from build123d import *

# Parameters (mm, degrees)
SKETCH004_R       = 5.031
PAD005_DEPTH      = 15
SKETCH007_W       = 23.03
SKETCH007_H       = 7
POCKET_DEPTH      = 9.031
POCKET_DEPTH_BACK = 9.031
SKETCH008_W       = 20
SKETCH008_H       = 23
PAD006_DEPTH      = 2
PAD012_DEPTH      = 4
PAD013_DEPTH      = 19


with BuildPart() as part:
    # Sketch004 → Pad005 (new body)
    with BuildSketch(Plane.XY):
        with BuildLine():
            ThreePointArc((-9.03, 0), (0, -9.03), (9.03, 0))
            Line((9.03, 0), (9.03, 16))
            Line((9.03, 16), (-9.03, 16))
            Line((-9.03, 16), (-9.03, 0))
        make_face()
        Circle(SKETCH004_R, mode=Mode.SUBTRACT)
    extrude(amount=PAD005_DEPTH)

    # Sketch007 → Pocket (cut, two sides)
    with BuildSketch(Plane.YZ) as pocket_sk:
        with Locations((2.485, 7.5)):
            Rectangle(SKETCH007_W, SKETCH007_H)
    extrude(amount=-POCKET_DEPTH, mode=Mode.SUBTRACT)
    extrude(pocket_sk.sketch, amount=POCKET_DEPTH_BACK, mode=Mode.SUBTRACT)

    # Sketch008 → Pad006 (join)
    with BuildSketch(Plane.XZ.offset(-16)):
        with Locations((10, 7.5)):
            Rectangle(SKETCH008_W, SKETCH008_H)
    extrude(amount=PAD006_DEPTH)

    # Sketch018 → Pad012 (join)
    with BuildSketch(Plane.XY):
        Polygon((14, 16.280637), (14, -8), (26, -8), (26, -4.5), (24, -4.5), (24, -6), (16, -6), (16, 14), (54, 14), (54, 12), (56, 12), (56, 14), (56, 16), (14, 16), align=None)
    extrude(amount=-PAD012_DEPTH)

    # Sketch018 → Pad013 (join)
    with BuildSketch(Plane.XY):
        Polygon((14, 16.280637), (14, -8), (26, -8), (26, -4.5), (24, -4.5), (24, -6), (16, -6), (16, 14), (54, 14), (54, 12), (56, 12), (56, 14), (56, 16), (14, 16), align=None)
    extrude(amount=PAD013_DEPTH)


solid = part.part
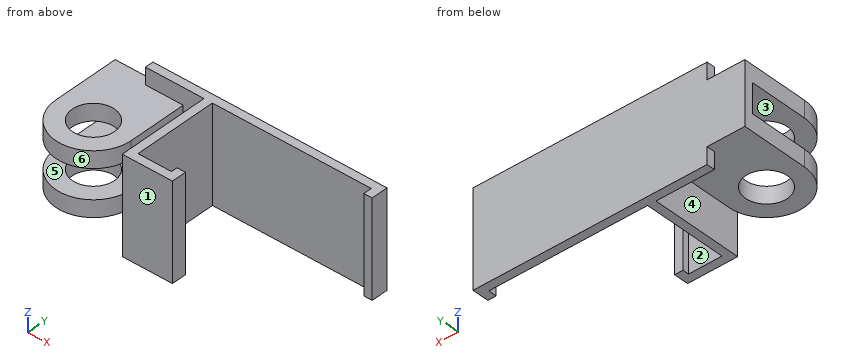
Check sheet for the modelled part. Datum: model origin and axes. Units: mm. Face numbers are marked on the shaded views. A direction names the side the tool comes from. Round coordinates to 2 decimals unless told otherwise and drop trailing zeros. Order: outer loops, then holes, each group sorted by start corner. A loop starts at its lowest first (then second) coordinate and runs counter-clockwise, first axis right, second up. Notation, with made-up numbers: M 63.5,-15.75 L 115.5,-15.75 A16 cw 115.5,-6.75 Z; hole C 6.25,22 d9. An arc over 180 degrees is marked long. One line per item, written item: value. Start each with the question number.
1. Section check D-D on x = 47.5. Enter the section's corners in (y, z), and give its area (3 significant figures).
2. Gauge pin test, flat ends, axial feed: P1, Ø1.6, axis at y = 15, z = -1.5, coming from the -X side; P2, Ø4, axis at y = -6.5, z = 10, coming from the +X side; P3, Ø14.5, axis at x = -3.5, y = 7, coming from the +Z side. Record the tip position at first contact, or that the pin passes through.
3. Scan lines: line 1 along X through (y, z) = (11, 12.5); line 2 along Y through (x, z) = (0, 12.15); line 3 along X through (y, z) = (0.75, 12). Record each from-to range of solid material in increasing order.
4. Access from +Z, -Z, +X, -X, +Y, -Y to the whole of each face (thin tool, end or side, straight path). Record for the marked faces 1, 2 and 3.
5. Section check C-C on y = -1. Enter the section's corners in (x, z).
6. Section check B-B on z = 14. Enter the section's corners in (x, y).
7. Release check for a two-part mould opening along X. For the marked faces 4, 5 and 6 record: released by +X, released by -X, zero draft, split by the parting line, or undercut.
8. Section check A-A on z = 7.5. Enter the section's corners in (x, y).
Results found:
1. outline: M 14,-4 L 16,-4 L 16,19 L 14,19 Z
1. area: 46.0 mm^2
2. P1: x = 0
2. P2: x = 26
2. P3: z = 15
3. line 1: -9.03 to 9.03, 14 to 16
3. line 2: -9.03 to -5.03, 5.03 to 16
3. line 3: -9.03 to -4.97, 4.97 to 9.03, 14 to 16
4. face 1: +Z, -Z, +X, -Y
4. face 2: +Z, -Z
4. face 3: -X, -Y
5. outline: M -8.97,0 L -4.93,0 L -4.93,4 L -8.97,4 Z; M -8.97,11 L -4.93,11 L -4.93,15 L -8.97,15 Z; M 4.93,0 L 8.97,0 L 8.97,4 L 4.93,4 Z; M 4.93,11 L 8.97,11 L 8.97,15 L 4.93,15 Z; M 14,-4 L 16,-4 L 16,19 L 14,19 Z
6. outline: M -9.03,0 A9.03 ccw 9.03,0 L 9.03,14 L 14,14 L 14,-8 L 26,-8 L 26,-4.5 L 24,-4.5 L 24,-6 L 16,-6 L 16,14 L 54,14 L 54,12 L 56,12 L 56,16 L -9.03,16 Z; hole C 0,0 d10.06
7. face 4: undercut
7. face 5: zero draft
7. face 6: undercut
8. outline: M -9.03,14 L 14,14 L 14,-8 L 26,-8 L 26,-4.5 L 24,-4.5 L 24,-6 L 16,-6 L 16,14 L 54,14 L 54,12 L 56,12 L 56,16 L -9.03,16 Z
